Read the model definition and answer for the solid it produces. Units are mm, in the model's axes. A direction names the side the tool comes from. Coordinates: 2 decimals unless noted, no trailing zeros. Write each loop counter-clockwise with the first axis right and the second up, starting at its lowest first coordinate (ties: lowest second). Pieces come first, ordered by that corner, then holes. Notation, with made-up numbers: (35.5, -12) -> (64.5, -12) arc R33 cw to (64.5, 26) -> close; hole circle Ø8 at (-16.75, 78). An arc over 180 degrees is marked (long way). One line per item, written item: value. Start each with the question number.
from build123d import *

# Parameters (mm, degrees)
BOSS_EXTRUDE1_DEPTH               = 300
F_3_0MM_DOWEL_HOLE1_D             = 3
F_3_0MM_DOWEL_HOLE2_D             = 3
SKETCH9_W                         = 1.5
SKETCH9_H                         = 1.999985051
F_3_0_3_DIAMETER_HOLE1_AT_2_COUNT = 2
F_3_0_3_DIAMETER_HOLE1_AT_2_PITCH = 24


with BuildPart() as part:
    # Sketch1 → Boss-Extrude1 (new body)
    with BuildSketch(Plane(origin=(0, 0, 0), x_dir=(1, 0, 0), z_dir=(0, 1, 0))):
        Polygon((0, 0), (0, 10), (2, 10), (2, 2), (20, 2), (20, 0), align=None)
    extrude(amount=BOSS_EXTRUDE1_DEPTH)

    # Ø3.0mm Dowel Hole1 (through all)
    with Locations(Plane.ZY):
        with Locations((-7.25, 2.75)):
            Hole(F_3_0MM_DOWEL_HOLE1_D / 2)

    # Ø3.0mm Dowel Hole2 (through all)
    with Locations(Plane.ZY):
        with Locations((-7.25, 211.25)):
            Hole(F_3_0MM_DOWEL_HOLE2_D / 2)

    # Sketch9 → Ø3.0 (3) Diameter Hole1 (revolve, cut)
    with BuildSketch(Plane(origin=(1.999985051, 288.000001132, -6.000000538), x_dir=(0, 0, -1), z_dir=(0, 1, 0))):
        with Locations((0.75, 0.999992526)):
            Rectangle(SKETCH9_W, SKETCH9_H)
    f_3_0_3_diameter_hole1 = revolve(axis=Axis((8.349985051, 288.000001132, -6.000000538), (-1, 0, 0)), mode=Mode.SUBTRACT)

    # Ø3.0 (3) Diameter Hole1 at 2: Ø3.0 (3) Diameter Hole1 ×2
    with Locations(*[(0, -i * F_3_0_3_DIAMETER_HOLE1_AT_2_PITCH, 0) for i in range(1, F_3_0_3_DIAMETER_HOLE1_AT_2_COUNT)]):
        add(f_3_0_3_diameter_hole1, mode=Mode.SUBTRACT)


solid = part.part
1. A cutting plane is placed at B-B on x = 7.5. Give the vertices of the cut face in (y, z), then the cut area to 3 significant figures.
2. A tool of negligible diameter and unlimited length cuts with its end or side. For faces 1 (the face through (7.1, 0, -1.7)), 2 (the face through (11, 148, -2)), from which of +Z, -Z, +X, -X, +Y, -Y can it reach the whole face along a straight path? Write none if from no direction.
3. A cutting plane is placed at A-A on y = 182. Give the vertices of the cut face in (x, z), then the cut area to 3 significant figures.
4. Find the intervals of material crossed by probe 1 along Y at (x, z) = (1.5, -7.25); probe 2 along Z at (x, y) = (1.15, 211.25); probe 3 along Y at (x, z) = (0.55, -6), in increasing order. Write a range as from..to.
5. Given pin 1 (2.5 mm diameter, centred on y = 288, z = -6, fed in from -X); pin 2 (2.5 mm diameter, centred on y = 264, z = -6, fed in from +X); pin 3 (5.5 mm diameter, centred on x = 6.5, y = 119.5, fed in from -Z), each flat-ended and moving along its own axis, determine where each tip first touches the part or whether it passes through.
Derived:
1. outline: (0, -2) -> (300, -2) -> (300, 0) -> (0, 0) -> close
1. area: 600 mm2
2. face 1: +Z, -Z, +X, -X, -Y
2. face 2: -Z, +X, +Y, -Y
3. outline: (0, -10) -> (2, -10) -> (2, -2) -> (20, -2) -> (20, 0) -> (0, 0) -> close
3. area: 56.0 mm2
4. probe 1: y = 0..1.25, 4.25..209.75, 212.75..263.17, 264.83..287.17, 288.83..300
4. probe 2: z = -10..-8.75, -5.75..0
4. probe 3: y = 0..1.92, 3.58..210.42, 212.08..262.5, 265.5..286.5, 289.5..300
5. pin 1: stops at x = 2
5. pin 2: stops at x = 2
5. pin 3: stops at z = -2
